Here's how the part is built. I have some questions about the finished solid (model axes, mm). Face numbers are marked on the shaded views. A direction names the side the tool comes from. Coordinates: 2 decimals unless noted, no trailing zeros. Write each loop counter-clockwise with the first axis right and the second up, starting at its lowest first coordinate (ties: lowest second). Pieces come first, ordered by that corner, then holes.
Item 1: I want a section at D-D (y = 5.75). Please give me the cut outline in (x, z) (1 decimal), and give its area (3 significant figures).
Item 2: I want a section at A-A (y = 11.25). Please give me the cut outline in (x, z) (1 decimal).
Item 3: For the marked faces 1, 2, 3, 4 and 5, which set-ups out of +Z, -Z, +X, -X, +Y, -Y let a thin tool reach every point of the face, with its end or its side?
Item 4: I'm going to push flat-ended pins straight in: P1, Ø3, axis at x = 10, z = -28.5, coming from the +Y side; P2, Ø3, axis at x = 4, z = -53.5, coming from the -Y side; P3, Ø1, axis at x = 9.5, y = 8.5, coming from the -Z side; P4, Ø3.5, axis at y = 5.5, z = -52, coming from the +X side. Where does each tip first touch, or does it pass through?
Item 5: Please list where these lines run through material, in increasing order: line 1 (Z direction, x = 3.75, y = 1.25); line 2 (Y direction, x = 12.5, z = -61.5); line 3 (X direction, y = 5, z = -69).
Item 6: I want a section at C-C (z = -66.5). Please give me the cut outline in (x, y) (1 decimal).
Item 7: If we mould it in two halves opening along Y, with no side actions, what happens to the marked faces 6, 7 and 8? For each: pulls with the +Y half, pulls with the -Y half, needs draft (parallel to the pull), parting line crosses it, or undercut.
Item 8: I want a section at B-B (x = 7). Please give me the cut outline in (y, z) (3 decimals).
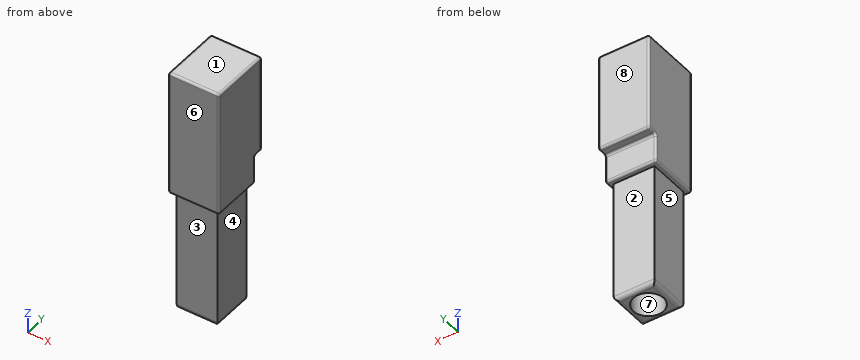
from build123d import *

# Parameters (mm, degrees)
BOSS_EXTRUDE1_DEPTH = 14.986
SKETCH2_W           = 12.065
SKETCH2_H           = 12.065
BOSS_EXTRUDE2_DEPTH = 36.322
FILLET1_R           = 1.27
FILLET2_R           = 0.635
SKETCH3_R           = 4.445
CUT_EXTRUDE1_DEPTH  = 31.75


with BuildPart() as part:
    # Sketch1 → Boss-Extrude1 (new body)
    with BuildSketch(Plane(origin=(0, 0, 0), x_dir=(0, 0, -1), z_dir=(1, 0, 0))):
        Polygon((0, 0), (0, 18.034), (28.956, 18.034), (28.956, 15.113), (37.338, 15.113), (37.338, 0), align=None)
    extrude(amount=BOSS_EXTRUDE1_DEPTH)

    # Sketch2 → Boss-Extrude2 (add)
    with BuildSketch(Plane(origin=(0, 0, -37.338), x_dir=(-1, 0, 0), z_dir=(0, 0, -1))):
        with Locations((-7.493, 7.5565)):
            Rectangle(SKETCH2_W, SKETCH2_H)
    extrude(amount=BOSS_EXTRUDE2_DEPTH)

    # Fillet1
    fillet1_edges = [part.edges().sort_by_distance(p)[0] for p in [
        (1.4605, 7.5565, -73.66),
        (7.493, 13.589, -73.66),
        (13.5255, 7.5565, -73.66),
        (7.493, 1.524, -73.66),
    ]]
    fillet(fillet1_edges, radius=FILLET1_R)

    # Fillet2
    fillet2_edges = [part.edges().sort_by_distance(p)[0] for p in [
        (14.986, 15.113, -33.147),
        (7.493, 0, 0),
        (7.493, 18.034, 0),
        (7.493, 18.034, -28.956),
        (7.493, 15.113, -28.956),
        (7.493, 15.113, -37.338),
        (7.493, 0, -37.338),
        (14.986, 16.5735, -28.956),
        (14.986, 18.034, -14.478),
        (14.986, 9.017, 0),
        (14.986, 0, -18.669),
        (0, 9.017, 0),
        (0, 18.034, -14.478),
        (0, 16.5735, -28.956),
        (14.986, 7.5565, -37.338),
        (0, 15.113, -33.147),
        (0, 7.5565, -37.338),
        (0, 0, -18.669),
    ]]
    fillet(fillet2_edges, radius=FILLET2_R)

    # Sketch3 → Cut-Extrude1 (cut)
    with BuildSketch(Plane(origin=(0, 0, -73.66), x_dir=(-1, 0, 0), z_dir=(0, 0, -1))):
        with Locations((-7.493, 7.5565)):
            Circle(SKETCH3_R)
    extrude(amount=-CUT_EXTRUDE1_DEPTH, mode=Mode.SUBTRACT)


solid = part.part
Answer:
1. outline: (0, -36.7) arc R0.6 ccw to (0.6, -37.3) - (1.5, -37.3) - (1.5, -72.4) arc R1.3 ccw to (2.7, -73.7) - (3.4, -73.7) - (3.4, -41.9) - (11.6, -41.9) - (11.6, -73.7) - (12.3, -73.7) arc R1.3 ccw to (13.5, -72.4) - (13.5, -37.3) - (14.4, -37.3) arc R0.6 ccw to (15, -36.7) - (15, -0.6) arc R0.6 ccw to (14.4, 0) - (0.6, 0) arc R0.6 ccw to (0, -0.6) - close
1. area: 739 mm2
2. outline: (0, -36.7) arc R0.6 ccw to (0.6, -37.3) - (1.5, -37.3) - (1.5, -72.4) arc R1.3 ccw to (2.7, -73.7) - (5, -73.7) - (5, -41.9) - (10, -41.9) - (10, -73.7) - (12.3, -73.7) arc R1.3 ccw to (13.5, -72.4) - (13.5, -37.3) - (14.4, -37.3) arc R0.6 ccw to (15, -36.7) - (15, -0.6) arc R0.6 ccw to (14.4, 0) - (0.6, 0) arc R0.6 ccw to (0, -0.6) - close
3. face 1: +Z, +X, -X, +Y, -Y
3. face 2: -Z, +X, -X, +Y
3. face 3: -Z, +X, -X, -Y
3. face 4: -Z, +X, +Y, -Y
3. face 5: -Z, -X, +Y, -Y
4. P1: stops at y = 18.03
4. P2: stops at y = 1.52
4. P3: stops at z = -41.91
4. P4: stops at x = 13.53
5. line 1: z = -37.34 to 0
5. line 2: y = 1.52 to 13.59
5. line 3: x = 1.46 to 3.86, 11.13 to 13.53
6. outline: (1.5, 1.5) - (13.5, 1.5) - (13.5, 13.6) - (1.5, 13.6) - close; hole circle Ø8.9 at (7.5, 7.6)
7. face 6: pulls with the -Y half
7. face 7: undercut
7. face 8: pulls with the +Y half
8. outline: (0, -36.703) arc R0.635 ccw to (0.635, -37.338) - (1.524, -37.338) - (1.524, -72.39) arc R1.27 ccw to (2.794, -73.66) - (3.139, -73.66) - (3.139, -41.91) - (11.974, -41.91) - (11.974, -73.66) - (12.319, -73.66) arc R1.27 ccw to (13.589, -72.39) - (13.589, -37.338) - (14.478, -37.338) arc R0.635 ccw to (15.113, -36.703) - (15.113, -29.591) arc R0.635 cw to (15.748, -28.956) - (17.399, -28.956) arc R0.635 ccw to (18.034, -28.321) - (18.034, -0.635) arc R0.635 ccw to (17.399, 0) - (0.635, 0) arc R0.635 ccw to (0, -0.635) - close
